Input: part model. Units: mm. Frame: model coordinates. Face numbers are marked on the shaded views. A direction names the side the tool comes from. Give positions to 0.01 mm unless a question says otherwise; leave off trailing zeros. Order: outer loops, then holes, each group sorted by start corner. A loop starts at its lowest first (then second) coordinate and runs counter-clockwise, first axis right, second up. Notation, with made-up numbers: (9.25, -6.75) - (29.25, -6.75) arc R36 cw to (29.25, 27.25) - close; hole circle Ø7 at (9, 43.5). An arc over 180 degrees is marked (long way). Use a Markdown table: item, result.
from build123d import *

# Parameters (mm, degrees)
RESSALTO_EXTRUS_O1_DEPTH          = 76
CORTE_EXTRUS_O2_DEPTH             = 91.309467661
RESSALTO_EXTRUS_O4_START          = -20
RESSALTO_EXTRUS_O4_DEPTH          = 20
CORTE_EXTRUS_O6_START             = -22
CORTE_EXTRUS_O6_DEPTH             = 16
ESBO_O12_R                        = 3.5
ESBO_O12_R_2                      = 1.6
CORTE_EXTRUS_O7_DEPTH             = 2
ESBO_O12_2_R                      = 1.6
CORTE_EXTRUS_O8_DEPTH             = 90.2814959
CORTE_EXTRUS_O8_DIRECTION_2_REACH = 91.281
RESSALTO_EXTRUS_O5_REACH          = 91.8
ESBO_O14_W                        = 6.792197014
ESBO_O14_H                        = 0.5
CASCA1_START                      = 1
CASCA1_DEPTH                      = 74
CASCA1_START_2                    = -3.278440116
CASCA1_2_OUTLINE_W                = 7
CASCA1_2_OUTLINE_H                = 18
CASCA1_2_OUTLINE_R                = 2.6
CASCA1_2_DEPTH                    = 1
CASCA1_START_3                    = -2.278440116
CASCA1_3_DEPTH                    = 1.5
RESSALTO_EXTRUS_O6_REACH          = 91.8
CORTE_EXTRUS_O9_DEPTH             = 91.309467661
CORTE_EXTRUS_O9_DEPTH_BACK        = 91.309467661
ESBO_O17_R                        = 1.6
RESSALTO_EXTRUS_O7_DEPTH          = 1


# Read off the part's stored shape, not the designer's step: Casca1
with BuildPart() as part:
    # Esboço1 → Ressalto-extrusão1 (new body)
    with BuildSketch(Plane.XY):
        with BuildLine():
            Line((-31.811733316, -8.523928252), (-26.064507457, -6.983963724))
            ThreePointArc((-26.064507457, -6.983963724), (-8.100799468, -10.557167407), (0, -26.983963724))
            Line((0, -26.983963724), (0, -36.983963724))
            Line((0, -36.983963724), (-14.5, -36.983963724))
            Line((-14.5, -36.983963724), (-14.5, -26.983963724))
            ThreePointArc((-14.5, -26.983963724), (-19.25882596, -17.334019289), (-29.811631303, -15.234935796))
            Line((-29.811631303, -15.234935796), (-30, -15.285409036))
            Line((-30, -15.285409036), (-31.811733316, -8.523928252))
        make_face()
    extrude(amount=RESSALTO_EXTRUS_O1_DEPTH)

    # Esboço3 → Corte-extrusão2 (cut, through all)
    with BuildSketch(Plane.XY.offset(76)):
        Polygon((-30.336464759, -14.029705462), (-30.336464759, -8.128631233), (-31.811733316, -8.523928252), align=None)
    extrude(amount=-CORTE_EXTRUS_O2_DEPTH, mode=Mode.SUBTRACT)

    # Esboço8 → Ressalto-extrusão4 (add)
    with BuildSketch(Plane(origin=(0, 0, 0), x_dir=(-1, 0, 0), z_dir=(0, 0, -1)).offset(RESSALTO_EXTRUS_O4_START)):
        with BuildLine():
            Line((9, -1.278440116), (5.9, -1.278440116))
            Line((5.9, -1.278440116), (5.9, 0.221559884))
            Line((5.9, 0.221559884), (3.1, 0.221559884))
            Line((3.1, 0.221559884), (3.1, -1.278440116))
            Line((3.1, -1.278440116), (0, -1.278440116))
            Line((0, -1.278440116), (0, -26.983963724))
            ThreePointArc((0, -26.983963724), (2.38766752, -17.331251347), (9, -9.90475341))
            Line((9, -9.90475341), (9, -1.278440116))
        make_face()
    extrude(amount=-RESSALTO_EXTRUS_O4_DEPTH)

    # Esboço8<3> → Corte-extrusão6 (cut)
    with BuildSketch(Plane(origin=(0, 0, 0), x_dir=(-1, 0, 0), z_dir=(0, 0, -1)).offset(CORTE_EXTRUS_O6_START)):
        with BuildLine():
            Line((9, -9.90475341), (9, -4.278440116))
            Line((9, -4.278440116), (0, -4.278440116))
            Line((0, -4.278440116), (0, -26.983963724))
            ThreePointArc((0, -26.983963724), (2.38766752, -17.331251347), (9, -9.90475341))
        make_face()
    extrude(amount=-CORTE_EXTRUS_O6_DEPTH, mode=Mode.SUBTRACT)

    # Esboço12 → Corte-extrusão7 (cut)
    with BuildSketch(Plane(origin=(0, -1.278440116, 0), x_dir=(1, 0, 0), z_dir=(0, 1, 0))):
        with Locations((-4.5, -30)):
            Circle(ESBO_O12_R)
        with Locations((-4.5, -30)):
            Circle(ESBO_O12_R_2, mode=Mode.SUBTRACT)
    extrude(amount=CORTE_EXTRUS_O7_DEPTH, mode=Mode.SUBTRACT)

    # Esboço12<2> → Corte-extrusão8 (cut)
    with BuildSketch(Plane(origin=(0, -1.278440116, 0), x_dir=(1, 0, 0), z_dir=(0, 1, 0))):
        with Locations(Location((-4.5, -30, 0), (0, 0, 180))):
            Circle(ESBO_O12_2_R)
    extrude(amount=CORTE_EXTRUS_O8_DEPTH, mode=Mode.SUBTRACT)

    # Esboço12<2> → Corte-extrusão8 direction 2 (cut, up to next)
    with BuildSketch(Plane(origin=(0, -1.278440116, 0), x_dir=(1, 0, 0), z_dir=(0, 1, 0)), mode=Mode.PRIVATE) as corte_extrus_o8_direction_2_sk1:
        with Locations(Location((-4.5, -30, 0), (0, 0, 180))):
            Circle(ESBO_O12_2_R)
    corte_extrus_o8_direction_2_tool1 = extrude(corte_extrus_o8_direction_2_sk1.sketch, amount=-CORTE_EXTRUS_O8_DIRECTION_2_REACH, mode=Mode.PRIVATE) & part.part
    add(corte_extrus_o8_direction_2_tool1.solids().sort_by_distance((-4.5, -1.27844, 30))[0], mode=Mode.SUBTRACT)

    # Esboço14 → Ressalto-extrusão5 (add, up to next)
    with BuildSketch(Plane(origin=(0, 0, 0), x_dir=(0, 0, -1), z_dir=(1, 0, 0)), mode=Mode.PRIVATE) as ressalto_extrus_o5_sk1:
        with Locations((-36.603901493, -0.028440116)):
            Rectangle(ESBO_O14_W, ESBO_O14_H)
    ressalto_extrus_o5_tool1 = extrude(ressalto_extrus_o5_sk1.sketch, amount=-RESSALTO_EXTRUS_O5_REACH, mode=Mode.PRIVATE) - part.part
    # Esboço14 → Ressalto-extrusão5 (add, up to next)
    with BuildSketch(Plane(origin=(0, 0, 0), x_dir=(0, 0, -1), z_dir=(1, 0, 0)), mode=Mode.PRIVATE) as ressalto_extrus_o5_sk2:
        with Locations((-23.396098507, -0.028440116)):
            Rectangle(ESBO_O14_W, ESBO_O14_H)
    ressalto_extrus_o5_tool2 = extrude(ressalto_extrus_o5_sk2.sketch, amount=-RESSALTO_EXTRUS_O5_REACH, mode=Mode.PRIVATE) - part.part
    add(ressalto_extrus_o5_tool1.solids().sort_by_distance((0, -0.02844, 36.603901))[0])
    add(ressalto_extrus_o5_tool2.solids().sort_by_distance((0, -0.02844, 23.396099))[0])

    # Casca1 outline → Casca1 (cut)
    with BuildSketch(Plane.XY.offset(CASCA1_START)):
        with BuildLine():
            Line((-25.805688412, -7.94988955), (-30.336464759, -9.163907414))
            Line((-30.336464759, -9.163907414), (-30.336464759, -14.029705462))
            Line((-30.336464759, -14.029705462), (-30.258819045, -14.31948321))
            Line((-30.258819045, -14.31948321), (-30.070450348, -14.269009969))
            ThreePointArc((-30.070450348, -14.269009969), (-18.650064531, -16.540665949), (-13.5, -26.983963724))
            Line((-13.5, -26.983963724), (-13.5, -36.983963724))
            Line((-13.5, -36.983963724), (-1, -36.983963724))
            Line((-1, -36.983963724), (-1, -26.983963724))
            ThreePointArc((-1, -26.983963724), (-8.709560897, -11.350520747), (-25.805688412, -7.94988955))
        make_face()
    extrude(amount=CASCA1_DEPTH, mode=Mode.SUBTRACT)

    # Casca1 2 outline → Casca1 2 (cut)
    with BuildSketch(Plane(origin=(0, 0, 0), x_dir=(1, 0, 0), z_dir=(0, 1, 0)).offset(CASCA1_START_2)):
        with Locations((-4.5, -30)):
            Rectangle(CASCA1_2_OUTLINE_W, CASCA1_2_OUTLINE_H)
        with Locations((-4.5, -30)):
            Circle(CASCA1_2_OUTLINE_R, mode=Mode.SUBTRACT)
    extrude(amount=CASCA1_2_DEPTH, mode=Mode.SUBTRACT)

    # Casca1 3 outline → Casca1 3 (cut)
    with BuildSketch(Plane(origin=(0, 0, 0), x_dir=(1, 0, 0), z_dir=(0, 1, 0)).offset(CASCA1_START_3)):
        with BuildLine():
            Line((-4.1, -25.517813034), (-4.1, -21))
            Line((-4.1, -21), (-4.9, -21))
            Line((-4.9, -21), (-4.9, -25.517813034))
            ThreePointArc((-4.9, -25.517813034), (-4.5, -25.5), (-4.1, -25.517813034))
        make_face()
        with BuildLine():
            Line((-4.9, -39), (-4.1, -39))
            Line((-4.1, -39), (-4.1, -34.482186966))
            ThreePointArc((-4.1, -34.482186966), (-4.5, -34.5), (-4.9, -34.482186966))
            Line((-4.9, -34.482186966), (-4.9, -39))
        make_face()
    extrude(amount=CASCA1_3_DEPTH, mode=Mode.SUBTRACT)

    # Esboço15 → Ressalto-extrusão6 (add, up to next)
    with BuildSketch(Plane(origin=(0, 0, 0), x_dir=(0.965925826289069, 0.2588190451025183, 0), z_dir=(-0.2588190451025183, 0.965925826289069, 0)), mode=Mode.PRIVATE) as ressalto_extrus_o6_sk1:
        Polygon((-32.933929759, -11), (-26.983963724, -15.561640627), (-26.983963724, -16.695704117), (-32.933929759, -12.13406349), align=None)
    ressalto_extrus_o6_tool1 = extrude(ressalto_extrus_o6_sk1.sketch, amount=-RESSALTO_EXTRUS_O6_REACH, mode=Mode.PRIVATE) - part.part
    # Esboço15 → Ressalto-extrusão6 (add, up to next)
    with BuildSketch(Plane(origin=(0, 0, 0), x_dir=(0.965925826289069, 0.2588190451025183, 0), z_dir=(-0.2588190451025183, 0.965925826289069, 0)), mode=Mode.PRIVATE) as ressalto_extrus_o6_sk2:
        Polygon((-32.933929759, -63.86593651), (-32.933929759, -65), (-26.983963724, -60.438359373), (-26.983963724, -59.304295883), align=None)
    ressalto_extrus_o6_tool2 = extrude(ressalto_extrus_o6_sk2.sketch, amount=-RESSALTO_EXTRUS_O6_REACH, mode=Mode.PRIVATE) - part.part
    add(ressalto_extrus_o6_tool1.solids().sort_by_distance((-28.93812, -7.753946, 13.847852))[0])
    add(ressalto_extrus_o6_tool2.solids().sort_by_distance((-28.93812, -7.753946, 62.152148))[0])

    # Esboço16 → Corte-extrusão9 (cut, two sides: drawn at the far end of the back side and taken through both)
    with BuildSketch(Plane.XY.offset(76).offset(-CORTE_EXTRUS_O9_DEPTH_BACK)):
        Polygon((-31.811733316, -8.523928252), (-30.336464759, -14.029705462), (-30.336464759, -8.128631233), align=None)
    extrude(amount=CORTE_EXTRUS_O9_DEPTH + CORTE_EXTRUS_O9_DEPTH_BACK, mode=Mode.SUBTRACT)

    # Esboço17 → Ressalto-extrusão7 (add)
    # profile 1 of 2: a face of its own
    with BuildSketch(Plane.ZY.offset(14.5)):
        with BuildLine():
            Line((0, -36.983963724), (-6.455184248, -44.800011084))
            ThreePointArc((-6.455184248, -44.800011084), (-5.78395264, -51.839147972), (1.255184248, -51.167916365))
            Line((1.255184248, -51.167916365), (12.969548739, -36.983963724))
            Line((12.969548739, -36.983963724), (0, -36.983963724))
        make_face()
        with Locations((-2.6, -47.983963724)):
            Circle(ESBO_O17_R, mode=Mode.SUBTRACT)
    # profile 2 of 2: a face of its own
    with BuildSketch(Plane.ZY.offset(14.5)):
        with BuildLine():
            Line((77.493198992, -39.1124272), (76, -36.983963724))
            Line((76, -36.983963724), (63.784615385, -36.983963724))
            Line((63.784615385, -36.983963724), (69.306801008, -44.855500248))
            ThreePointArc((69.306801008, -44.855500248), (76.271536524, -46.077162717), (77.493198992, -39.1124272))
        make_face()
        with Locations((73.4, -41.983963724)):
            Circle(ESBO_O17_R, mode=Mode.SUBTRACT)
    extrude(amount=-RESSALTO_EXTRUS_O7_DEPTH)


solid = part.part
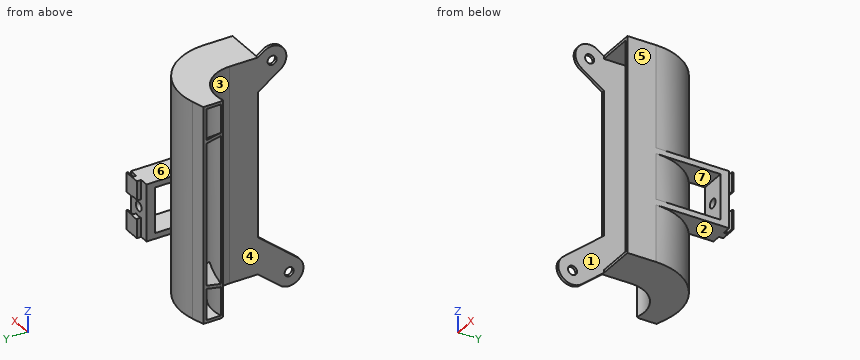
1. Section query C-C (y = -17). Return loops of the section in (x, z).
Response:
| item | result |
|---|---|
| outline | (-19.72, 0) - (-2.57, 0) - (-2.57, 20) - (0, 20) - (0, 22) - (-2.57, 22) - (-2.57, 38) - (0, 38) - (0, 40) - (-2.57, 40) - (-2.57, 76) - (-19.72, 76) - close; hole (-18.08, 1) - (-3.72, 1) - (-3.72, 75) - (-18.08, 75) - close |
2. Section query D-D (z = 6). Return loops of the section in (x, y).
Response:
| item | result |
|---|---|
| outline | (-30.34, -9.16) - (-25.81, -7.95) arc R19.71 cw to (-1, -26.98) - (-1, -36.98) - (0, -36.98) - (0, -26.98) arc R20.71 ccw to (-26.06, -6.98) - (-30.34, -8.13) - close; (-30.26, -14.32) - (-30, -15.29) - (-29.81, -15.23) arc R12.16 cw to (-14.5, -26.98) - (-14.5, -45.42) - (-13.5, -45.42) - (-13.5, -26.98) arc R13.16 ccw to (-30.07, -14.27) - close |
3. Material intervals for line 1 along Z through (x, y) = (-4.5, -2.45); line 2 along Z through (x, y) = (-10.5, -29); line 3 along X through (y, z) = (-36, 68), sorted ascending.
Response:
| item | result |
|---|---|
| line 1 | z = 20 to 21, 27.4 to 28.4, 31.6 to 32.6, 39 to 40 |
| line 2 | z = 0 to 1, 75 to 76 |
| line 3 | x = -14.5 to -13.5, -1 to 0 |
4. Section query A-A (z = 30). State how many separate pieces and enclosed holes the cut face has, then the cut area to 3 significant figures.
Response:
| item | result |
|---|---|
| separate pieces | 4 |
| enclosed holes | 2 |
| area | 101 mm^2 |
5. Mould query, pull axis X, two halves, no side actions, for the marked faces 1, 2, 3 and 4. Classes: pulls with the +X half, pulls with the -X half, needs draft (parallel to the pull), parting line crosses it, or undercut.
Response:
| item | result |
|---|---|
| face 1 | undercut |
| face 2 | needs draft |
| face 3 | undercut |
| face 4 | pulls with the -X half |
6. Section query B-B (z = 73.4). Return loops of the section in (x, y).
Response:
| item | result |
|---|---|
| outline | (-30.34, -9.16) - (-25.81, -7.95) arc R19.71 cw to (-1, -26.98) - (-1, -36.98) - (0, -36.98) - (0, -26.98) arc R20.71 ccw to (-26.06, -6.98) - (-30.34, -8.13) - close; (-30.26, -14.32) - (-30, -15.29) - (-29.81, -15.23) arc R12.16 cw to (-14.5, -26.98) - (-14.5, -40.38) - (-13.5, -40.38) - (-13.5, -26.98) arc R13.16 ccw to (-30.07, -14.27) - close; (-14.5, -46.98) - (-13.5, -46.98) - (-13.5, -43.58) - (-14.5, -43.58) - close |
7. Set-up query: the marked faces 5, 6 and 7. Return all of +Z, -Z, +X, -X, +Y, -Y with unobstructed straight access to the full face (end or side cutting, diameter ignored); none if empty.
Response:
| item | result |
|---|---|
| face 5 | +Z, -Z, +X, +Y, -Y |
| face 6 | +Z, +X, +Y |
| face 7 | +X |
8. Pin query (flat end, axial travel): pin 1 (3 mm diameter, centred on y = -6.5, z = 44.5, fed in from +X); pin 2 (8 mm diameter, centred on y = -37.5, z = 42.5, fed in from -X); pin 3 (15 mm diameter, centred on x = -14, y = -15.5, fed in from +Z). Return the tip coordinate at first contact, or that it passes through.
Response:
| item | result |
|---|---|
| pin 1 | stops at x = -12.44 |
| pin 2 | stops at x = -14.5 |
| pin 3 | stops at z = 76 |
